Design review of the part built by this model. Coordinates are the model's own, in mm. Give positions to 0.01 mm unless a question says otherwise; leave off trailing zeros. Order: outer loops, then holes, each group sorted by start corner. A loop starts at its lowest first (then second) coordinate and runs counter-clockwise, first axis right, second up. Notation, with made-up numbers: (14.5, 2) -> (29.5, 2) arc R13 ccw to (29.5, 25) -> close; hole circle Ø5 at (71.5, 55.5). An arc over 180 degrees is marked (long way). Answer in a Markdown table with one row per item. Add a question column.
```python
from build123d import *

# Parameters (mm, degrees)
F0_W     = 50
F0_H     = 50
F0_R     = 2.5
F0_R_2   = 19
F0_W_2   = 40
F1_DEPTH = 12
F2_R     = 1.4
F3_DEPTH = 12.001
F4_R     = 5


with BuildPart() as f1:
    # F0 (on Top) → F1 (new body)
    with BuildSketch(Plane.XY):
        Rectangle(F0_W, F0_H)
        with Locations((-16.970563, -16.970563)):
            Circle(F0_R, mode=Mode.SUBTRACT)
        with Locations((16.970563, -16.970563)):
            Circle(F0_R, mode=Mode.SUBTRACT)
        Circle(F0_R_2, mode=Mode.SUBTRACT)
        with Locations((-16.970563, 16.970563)):
            Circle(F0_R, mode=Mode.SUBTRACT)
        with Locations((16.970563, 16.970563)):
            Circle(F0_R, mode=Mode.SUBTRACT)
        with Locations((45, 0)):
            Rectangle(F0_W_2, F0_H)
        with Locations((50, -15)):
            Circle(F0_R, mode=Mode.SUBTRACT)
        with Locations((50, 15)):
            Circle(F0_R, mode=Mode.SUBTRACT)
    extrude(amount=F1_DEPTH)

    # F2 (on face) → F3 (cut, through all)
    with BuildSketch(Plane.XY.offset(12)):
        with Locations((0, 22)):
            Circle(F2_R)
    extrude(amount=-F3_DEPTH, mode=Mode.SUBTRACT)

    # F4
    f4_edges = [f1.edges().sort_by_distance(p)[0] for p in [
        (65, -25, 6),
        (-25, -25, 6),
        (-25, 25, 6),
        (65, 25, 6),
    ]]
    fillet(f4_edges, radius=F4_R)


solid = f1.part
```
1) Add section B-B, the plane y = 0. Write out the cut boundary in (x, z).
2) Mouldability with a two-part tool opening along Y and no side actions: class faces 1 (the face through (8.767, -16.856, 5.916)), 2 (the face through (65, 0, 6)), 3 (the face through (63, 24, 6)) as +Y half, -Y half, draft (parallel to the pull), parting line (faces both ways), or undercut.
3) Add section C-C, the plane x = 10.5. Write out the cut boundary in (y, z).
4) Add section D-D, the plane z = 5.25. Give the number of separate pieces and of enclosed holes in the cut face, and give its area (3 significant figures).
5) For L1, parallel to Y at x = 50, z = 5.75; L2, parallel to Y at x = 12.5, z = 8; L3, parallel to Y at x = 51, z = 6.25, list the stretches that pass through material, from the lowest coordinate up.
6) Add section A-A, the plane x = 50. Write out the cut boundary in (y, z).
Verdict:
| question | item | result |
|---|---|---|
| 1 | outline | (-25, 0) -> (-19, 0) -> (-19, 12) -> (-25, 12) -> close; (19, 0) -> (65, 0) -> (65, 12) -> (19, 12) -> close |
| 2 | face 1 | undercut |
| 2 | face 2 | draft |
| 2 | face 3 | +Y half |
| 3 | outline | (-25, 0) -> (-15.84, 0) -> (-15.84, 12) -> (-25, 12) -> close; (15.84, 0) -> (25, 0) -> (25, 12) -> (15.84, 12) -> close |
| 4 | separate pieces | 1 |
| 4 | enclosed holes | 8 |
| 4 | area | 3,220 mm2 |
| 5 | L1 | y = -25 to -17.5, -12.5 to 12.5, 17.5 to 25 |
| 5 | L2 | y = -25 to -14.31, 14.31 to 25 |
| 5 | L3 | y = -25 to -17.29, -12.71 to 12.71, 17.29 to 25 |
| 6 | outline | (-25, 0) -> (-17.5, 0) -> (-17.5, 12) -> (-25, 12) -> close; (-12.5, 0) -> (12.5, 0) -> (12.5, 12) -> (-12.5, 12) -> close; (17.5, 0) -> (25, 0) -> (25, 12) -> (17.5, 12) -> close |
